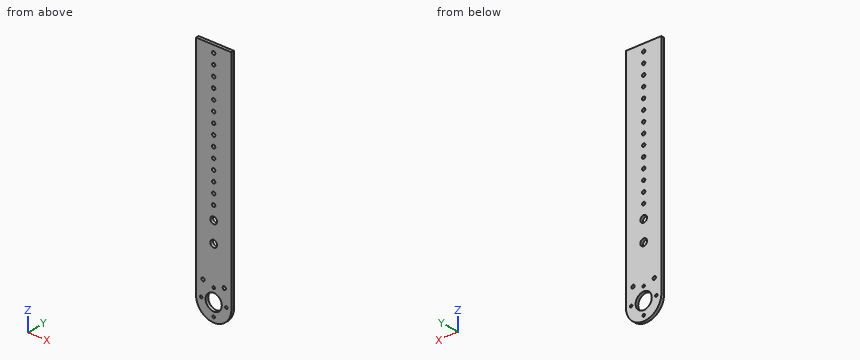
Autodesk Inventor part; units mm, degrees
ref_plane "YZ Plane" through (0, 0, 0) normal (1, 0, 0) x (0, 1, 0)
ref_plane "XZ Plane" through (0, 0, 0) normal (0, 1, 0) x (-1, 0, 0)
ref_plane "XY Plane" through (0, 0, 0) normal (0, 0, 1) x (1, 0, 0)
sketch "スケッチ1" plane through (0, 0, 0) normal (0, 1, 0) x (-1, 0, 0)
  line L0 (0, 0) -> (-35, 0)
  line L1 (-35, 0) -> (-35, -220)
  line L2 (-35, -220) -> (0, -220)
  line L3 (0, -220) -> (0, 0)
  arc A0 (-35, -220) -> (0, -220) centre (-17.5, -220) ccw
  dimension "d0" = 35
  dimension "d1" = 220
  dimension "d2" = 17.5
extrude "押し出し1" add sketch "スケッチ1" along normal blind 3
sketch "スケッチ2" plane through (0, 3, 0) normal (0, 1, 0) x (1, 0, 0)
  line L0 (0, 0) -> (35, 0) construction
  line L1 (17.5, 0) -> (17.5, 237.5) construction
  arc A0 (35, 220) -> (0, 220) centre (17.5, 220) ccw construction
hole "穴1" at (17.5, 3, -220) direction (0, -1, 0) diameter 16 end through all
sketch "スケッチ3" plane through (0, 3, 0) normal (0, 1, 0) x (1, 0, 0)
  circle A0 centre (17.5, 220) radius 8
  circle A1 centre (17.5, 220) radius 12.5
  point P0 (0, 0)
  point P1 (5, 220)
  point P2 (30, 220)
  point P3 (17.5, 232.5)
  point P4 (17.5, 207.5)
  dimension "d12" = 25
hole "穴2" at (5, 3, -220) at (30, 3, -220) at (17.5, 3, -232.5) at (17.5, 3, -207.5) direction (0, -1, 0) diameter 2.459 end through all
sketch "スケッチ4" plane through (0, 3, 0) normal (0, 1, 0) x (1, 0, 0)
  line L0 (0, 0) -> (35, 0) construction
  line L1 (17.5, 0) -> (17.5, 237.5) construction
  arc A0 (35, 220) -> (0, 220) centre (17.5, 220) ccw construction
  circle A1 centre (17.5, 220) radius 8
  point P0 (17.5, 137)
  point P1 (17.5, 127)
  point P2 (17.5, 117)
  point P3 (17.5, 107)
  point P4 (17.5, 97)
  point P5 (17.5, 87)
  point P6 (17.5, 77)
  point P7 (17.5, 67)
  point P8 (17.5, 57)
  point P9 (17.5, 47)
  point P10 (17.5, 37)
  point P11 (17.5, 27)
  point P12 (17.5, 17)
  point P13 (17.5, 7)
  dimension "d42" = 83
  dimension "d45" = 10
hole "穴3" at (17.5, 3, -137) at (17.5, 3, -127) at (17.5, 3, -117) at (17.5, 3, -107) at (17.5, 3, -97) at (17.5, 3, -87) at (17.5, 3, -77) at (17.5, 3, -67) at (17.5, 3, -57) at (17.5, 3, -47) at (17.5, 3, -37) at (17.5, 3, -27) at (17.5, 3, -17) at (17.5, 3, -7) direction (0, -1, 0) diameter 3.2 end through all
sketch "スケッチ5" plane through (0, 3, 0) normal (0, 1, 0) x (1, 0, 0)
  line L0 (0, 0) -> (35, 0) construction
  line L1 (17.5, 0) -> (17.5, 237.5) construction
  arc A0 (35, 220) -> (0, 220) centre (17.5, 220) ccw construction
  circle A1 centre (17.5, 137) radius 1.6 construction
  point P0 (17.5, 150)
  point P1 (17.5, 170)
  dimension "d50" = 13
  dimension "d51" = 20
hole "穴4" at (17.5, 3, -150) at (17.5, 3, -170) direction (0, -1, 0) diameter 6.6 end through all
sketch "スケッチ6" plane through (0, 3, 0) normal (0, 1, 0) x (1, 0, 0)
  line L0 (35, 0) -> (35, 220)
  line L1 (35, 204.2) -> (0, 204.2) construction
  line L2 (0, 220) -> (0, 0)
  circle A0 centre (17.5, 220) radius 8
  line L3 (17.5, 220) -> (17.5, 204.2) construction
  point P0 (28, 204.2)
  point P1 (7, 204.2)
  dimension "d52" = 15.8
  dimension "d53" = 10.5
  dimension "d54" = 10.5
hole "穴5" at (28, 3, -204.2) at (7, 3, -204.2) direction (0, -1, 0) diameter 3.3 end through all
properties part number "shoulder2_upper_plate_rigth" material "アルミニウム 5052"
Model file for the job. Use its own axes, mm. Round coordinates to 2 decimals unless told otherwise and drop trailing zeros. Answer as CSV lines item,"result". Start each with the question number.
1) Pin check, flat tip, straight feed: P1, Ø3, axis at x = 17.5, z = -207.5, coming from the +Y side. Stop position of the tip, or through.
2) Slice it at A-A (y = 1). State how many separate pieces and enclosed holes the cut face has, plus the area to 3 significant figures.
3) Probe line 1 along X through (y, z) = (2, -67); line 2 along Z through (x, y) = (5.5, 1.95); line 3 along X through (y, z) = (1.6, -207.5). List the from-to ranges inside material, lowest first.
Filled in:
1,P1,"stops at y = 3"
2,separate pieces,"1"
2,enclosed holes,"23"
2,area,"7,760 mm2"
3,line 1,"x = 0 to 15.9, 19.1 to 35"
3,line 2,"z = -232.74 to -221.12, -218.88 to -204.89, -203.51 to 0"
3,line 3,"x = 0 to 16.27, 18.73 to 35"
